The listing builds one solid part. Answer for the finished solid, in the listing's coordinates (mm). Round coordinates to 2 decimals unless told otherwise and drop trailing zeros. Write each loop counter-clockwise with the first axis right and the second up, starting at its lowest first coordinate (ties: lowest second). Pieces come first, ordered by that corner, then holes.
(1) Each of these flat-tipped pins is pushed along its axis until it touches: pin 1 Ø1 at (y, z) = (1.5, -32) entering from +X; pin 2 Ø1.8 at (x, y) = (-10, 3) entering from +Z; pin 3 Ø1.8 at (x, y) = (-16.5, 4) entering from -Z. Where does it stop, or does it pass through?
(2) Find the intervals of material crossed by probe 1 along Z at (x, y) = (-16, 4.7) (3 decimals); probe 2 along Z at (x, y) = (-57.25, 1.45); probe 3 along X at (y, z) = (0.65, -4), in increasing order.
(3) A cutting plane is placed at C-C, the plane x = -7. Give the vertices of the cut face in (y, z).
(4) A cutting plane is placed at D-D, the plane z = -24. Give the vertices of the cut face in (x, y).
(5) A cutting plane is placed at B-B, the plane z = 15.25. Give the vertices of the cut face in (x, y), and give its area (3 significant figures).
(6) A cutting plane is placed at A-A, the plane x = -16. Give the vertices of the cut face in (y, z) (3 decimals), and give its area (3 significant figures).
Autodesk Inventor part; units mm, degrees
ref_plane "YZ Plane" through (0, 0, 0) normal (1, 0, 0) x (0, 1, 0)
ref_plane "XZ Plane" through (0, 0, 0) normal (0, 1, 0) x (-1, 0, 0)
ref_plane "XY Plane" through (0, 0, 0) normal (0, 0, 1) x (1, 0, 0)
sketch "Sketch1" plane through (0, 0, 0) normal (0, 1, 0) x (-1, 0, 0)
  line L0 (0, 0) -> (0, -19)
  line L1 (0, 0) -> (0, 19)
  line L2 (0, 0) -> (19, 0) construction
  line L3 (0, 19) -> (32, 19)
  line L4 (0, -19) -> (32, -19)
  line L5 (68.5, 0) -> (68.5, -35)
  line L6 (68.5, 0) -> (68.5, 35)
  circle A0 centre (16, 0) radius 6.5
  circle A1 centre (25.125, 0) radius 1.75
  line L7 (55, -30) -> (44.25, -30)
  line L8 (44.25, -30) -> (44.25, 12)
  line L9 (44.25, 12) -> (65.5, 12)
  line L10 (65.5, 12) -> (65.5, 0)
  line L11 (65.5, 0) -> (65.5, -30)
  line L12 (65.5, -30) -> (55, -30)
  line L13 (68.5, -30) -> (68.5, -32)
  circle A2 centre (60.25, -33.25) radius 1.25
  circle A3 centre (50.25, -33.25) radius 1.25
  circle A4 centre (60.25, 15.25) radius 1.25
  circle A5 centre (50.25, 15.25) radius 1.25
  circle A6 centre (16, 9.125) radius 1.75
  circle A7 centre (6.875, 0) radius 1.75
  circle A8 centre (16, -9.125) radius 1.75
  line L14 (68.5, 0) -> (65.5, 0)
  circle A9 centre (57.25, -45.25) radius 1.75
  line L15 (55.5, -45.25) -> (49.3011, -45.25)
  arc A10 (51.25, -45.25) -> (63.25, -45.25) centre (57.25, -45.25) ccw
  line L16 (51.25, -45.25) -> (32, -19)
  line L17 (63.25, -41.5) -> (63.25, -45.25)
  line L18 (68.5, -35) -> (63.25, -41.5)
  circle A11 centre (57.25, 45.25) radius 1.75
  arc A12 (63.25, 45.25) -> (51.25, 45.25) centre (57.25, 45.25) ccw
  line L19 (51.25, 45.25) -> (32, 19)
  line L20 (63.25, 41.5) -> (63.25, 45.25)
  line L21 (68.5, 35) -> (63.25, 41.5)
  circle A13 centre (55.5, 19.25) radius 1.25
  dimension "d0" = 19
  dimension "d1" = 19
  dimension "d2" = 90
  dimension "d3" = 32
  dimension "d4" = 68.5
  dimension "d5" = 35
  dimension "d8" = 13
  dimension "d10" = 3.5
  dimension "d18" = 10.75
  dimension "d22" = 2.5
  dimension "d30" = 360
  dimension "d35" = 12
extrude "Extrusion1" add sketch "Sketch1" along normal blind 6
properties part number "Claw_Main"
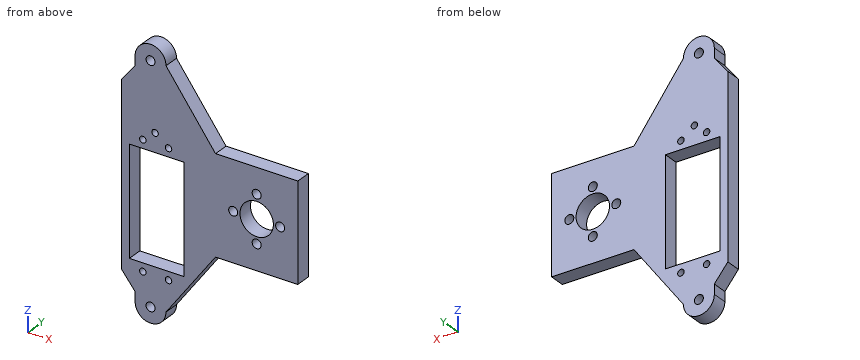
Solutions:
1. pin 1: stops at x = -41.17
1. pin 2: stops at z = 19
1. pin 3: stops at z = -19
2. probe 1: z = -19 to -10.875, -7.375 to -6.5, 6.5 to 7.375, 10.875 to 19
2. probe 2: z = -51.25 to -47, -43.5 to -30, 12 to 43.5, 47 to 51.25
2. probe 3: x = -68.5 to -65.5, -44.25 to -21.12, -10.88 to 0
3. outline: (0, -19) - (6, -19) - (6, -1.75) - (0, -1.75) - close; (0, 1.75) - (6, 1.75) - (6, 19) - (0, 19) - close
4. outline: (-68.5, 0) - (-65.5, 0) - (-65.5, 6) - (-68.5, 6) - close; (-44.25, 0) - (-35.67, 0) - (-35.67, 6) - (-44.25, 6) - close
5. outline: (-68.5, 0) - (-61.5, 0) - (-61.5, 6) - (-68.5, 6) - close; (-59, 0) - (-51.5, 0) - (-51.5, 6) - (-59, 6) - close; (-49, 0) - (0, 0) - (0, 6) - (-49, 6) - close
5. area: 381 mm2
6. outline: (0, -19) - (6, -19) - (6, -10.875) - (0, -10.875) - close; (0, -7.375) - (6, -7.375) - (6, -6.5) - (0, -6.5) - close; (0, 6.5) - (6, 6.5) - (6, 7.375) - (0, 7.375) - close; (0, 10.875) - (6, 10.875) - (6, 19) - (0, 19) - close
6. area: 108 mm2
